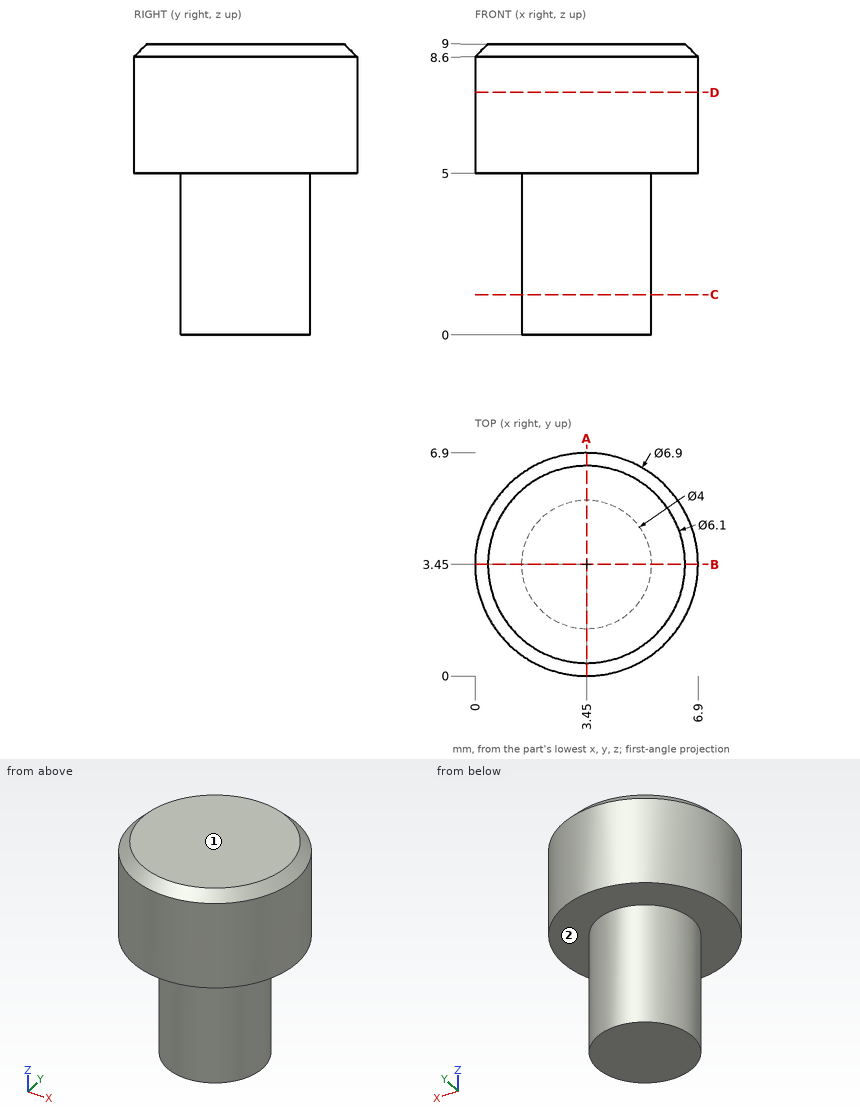
Could you check a few things on this drawing? It's one solid part, dimensions in mm from its lowest x, y, z. A direction names the side the tool comes from. Coordinates: 2 decimals unless noted, no trailing zeros. Loops run counter-clockwise (first coordinate to the right, second up) from the corner with the lowest first, then second, coordinate; pieces in that order, holes last.
1. I need wall thicknesses on L1, parallel to Z at x = 4, y = 0.5; L2, parallel to X at y = 4.5, z = 0.5; L3, parallel to Y at x = 4.25, z = 3.25. Which ranges of each line are inside material? Lowest first, please.
2. Imagine slicing it at C-C (z = 1.25). Please give me the cut outline in (x, y).
3. Imagine slicing it at A-A (x = 3.45). Please give me the cut outline in (y, z), and give its area (3 significant figures).
4. For the marked faces 1 and 2, which set-ups out of +Z, -Z, +X, -X, +Y, -Y let a thin tool reach every point of the face, with its end or its side?
5. Imagine slicing it at D-D (z = 7.5). Please give me the cut outline in (x, y).
6. For P1, Ø3, axis at y = 4.5, z = 2, coming from the +X side; P2, Ø3, axis at x = 5.5, z = 5, coming from the +Y side; P3, Ø2, axis at x = 1.5, z = 2.5, coming from the +Y side, each with a flat end and sliding along its axis, tell me the tip position at first contact or that it passes through.
Computed values:
1. L1: z = 5 to 9
1. L2: x = 1.75 to 5.15
1. L3: y = 1.62 to 5.28
2. outline: circle Ø4 at (3.45, 3.45)
3. outline: (0, 5) - (1.45, 5) - (1.45, 0) - (5.45, 0) - (5.45, 5) - (6.9, 5) - (6.9, 8.6) - (6.5, 9) - (0.4, 9) - (0, 8.6) - close
3. area: 47.4 mm2
4. face 1: +Z, +X, -X, +Y, -Y
4. face 2: -Z
5. outline: circle Ø6.9 at (3.45, 3.45)
6. P1: stops at x = 5.45
6. P2: stops at y = 6.86
6. P3: stops at y = 5.21
